from build123d import *

# Parameters (mm, degrees)
F0_W     = 76.2
F0_H     = 76.2
F1_DEPTH = 533.4
F2_R     = 9.525
F3_DEPTH = 101.6
F4_W     = 19.05
F4_H     = 38.1
F5_DEPTH = 76.2
F6_W     = 19.05
F6_H     = 19.05
F7_DEPTH = 76.201
F8_R     = 12.7


with BuildPart() as f1:
    # F0 (on Top) → F1 (new body)
    with BuildSketch(Plane.XY):
        Rectangle(F0_W, F0_H)
    extrude(amount=F1_DEPTH)

    # F2 (on face) → F3 (cut)
    with BuildSketch(Plane.XY.offset(533.4)):
        Circle(F2_R)
    extrude(amount=-F3_DEPTH, mode=Mode.SUBTRACT)

    # F4 (on face) → F5 (cut, through all)
    with BuildSketch(Plane.XZ.offset(38.1)):
        with Locations((0, 38.1)):
            Rectangle(F4_W, F4_H)
    extrude(amount=-F5_DEPTH, mode=Mode.SUBTRACT)

    # F6 (on face) → F7 (cut, through all)
    with BuildSketch(Plane.YZ.offset(38.1)):
        with Locations((0, 38.1)):
            Rectangle(F6_W, F6_H)
    extrude(amount=-F7_DEPTH, mode=Mode.SUBTRACT)

    # F8
    f8_edges = [f1.edges().sort_by_distance(p)[0] for p in [
        (-38.1, -38.1, 266.7),
        (38.1, -38.1, 266.7),
        (38.1, 38.1, 266.7),
        (-38.1, 38.1, 266.7),
    ]]
    fillet(f8_edges, radius=F8_R)


solid = f1.part
For this review, take the finished solid that the model builds, in its own axes (mm). A direction names the side the tool comes from. Coordinates: 2 decimals unless noted, no trailing zeros. Loops run counter-clockwise (first coordinate to the right, second up) from the corner with the lowest first, then second, coordinate; pieces in that order, holes last. Notation, with made-up numbers: (78.5, 61) - (99.5, 61) arc R15 cw to (99.5, 87) - close; hole circle Ø3 at (-11, 51). An arc over 180 degrees is marked (long way). Use a Markdown table: item, result. Add a question column.
Item 1: We need section B-B (x = 0). Give the boundary of the cut face in (y, z) (3 decimals).
Item 2: For line 1 (Z direction, x = -1.5, y = -8.5); line 2 (Y direction, x = 0, z = 511.5) (3 decimals); line 3 (Z direction, x = -2, y = 17), list the stretches that pass through material, from the lowest coordinate up.
Item 3: Mouldability with a two-part tool opening along Y and no side actions: class faces 6 (the face through (0, 0, 431.8)), 7 (the face through (-9.525, -1, 25)), 8 (the face through (-34.48, -34.28, 270.43)), 9 (the face through (24, 9.525, 38)) as pulls with the +Y half, pulls with the -Y half, needs draft (parallel to the pull), parting line crosses it, or undercut.
Item 4: We need section C-C (y = -19). Give the boundary of the cut face in (x, z) (3 decimals).
Item 5: Tool access review of faces 1 (the face through (-7.559, -5.796, 483.311)), 2 (the face through (34.28, -34.48, 270.43)), 3 (the face through (24, -9.525, 38)), 4 (the face through (0, -38.1, 263)), 5 (the face through (0, -1, 57.15)): name each direction out of +Z, -Z, +X, -X, +Y, -Y from which nothing blocks a thin tool from reaching the whole face with its end or side.
Item 6: We need section A-A (z = 440). Give the boundary of the cut face in (x, y) (3 decimals).
Item 7: Insertion check: pin 1 Ø17 at (x, y) = (0, 0) entering from +Z; pin 2 Ø4 at (x, z) = (29.5, 460) entering from +Y. Each pin has a flat end and moves straight along its axis. Give the tip position at first contact, or say it passes through.
Item 8: We need section D-D (z = 158). Give the boundary of the cut face in (x, y), and give its area (3 significant figures).
Results list:
| question | item | result |
|---|---|---|
| 1 | outline | (-38.1, 0) - (38.1, 0) - (38.1, 19.05) - (-38.1, 19.05) - close; (-38.1, 57.15) - (38.1, 57.15) - (38.1, 533.4) - (9.525, 533.4) - (9.525, 431.8) - (-9.525, 431.8) - (-9.525, 533.4) - (-38.1, 533.4) - close |
| 2 | line 1 | z = 0 to 19.05, 57.15 to 431.8 |
| 2 | line 2 | y = -38.1 to -9.525, 9.525 to 38.1 |
| 2 | line 3 | z = 0 to 19.05, 57.15 to 533.4 |
| 3 | face 6 | undercut |
| 3 | face 7 | needs draft |
| 3 | face 8 | pulls with the -Y half |
| 3 | face 9 | undercut |
| 4 | outline | (-38.1, 0) - (38.1, 0) - (38.1, 533.4) - (-38.1, 533.4) - close; hole (-9.525, 19.05) - (9.525, 19.05) - (9.525, 57.15) - (-9.525, 57.15) - close |
| 5 | face 1 | +Z |
| 5 | face 2 | +Z, -Z, +X, -Y |
| 5 | face 3 | +X, -X |
| 5 | face 4 | +Z, -Z, +X, -X, -Y |
| 5 | face 5 | +Y, -Y |
| 6 | outline | (-38.1, -25.4) arc R12.7 ccw to (-25.4, -38.1) - (25.4, -38.1) arc R12.7 ccw to (38.1, -25.4) - (38.1, 25.4) arc R12.7 ccw to (25.4, 38.1) - (-25.4, 38.1) arc R12.7 ccw to (-38.1, 25.4) - close; hole circle Ø19.05 at (0, 0) |
| 7 | pin 1 | stops at z = 431.8 |
| 7 | pin 2 | stops at y = 37.93 |
| 8 | outline | (-38.1, -25.4) arc R12.7 ccw to (-25.4, -38.1) - (25.4, -38.1) arc R12.7 ccw to (38.1, -25.4) - (38.1, 25.4) arc R12.7 ccw to (25.4, 38.1) - (-25.4, 38.1) arc R12.7 ccw to (-38.1, 25.4) - close |
| 8 | area | 5,670 mm^2 |
